CAD build for the part. Positions are in the model's coordinates, mm. A direction names the side the tool comes from. Coordinates: 2 decimals unless noted, no trailing zeros. Order: outer loops, then holes, each group sorted by start corner. A loop starts at its lowest first (then second) coordinate and runs counter-clockwise, first axis right, second up. Notation, with made-up numbers: M -5.5,-37.75 L 31.5,-37.75 A23 cw 31.5,-25.75 Z; hole C 37.25,38.25 d8. An arc over 180 degrees is marked long. Write item = value, one per line.
Autodesk Inventor part; units mm, degrees
ref_plane "YZ Plane" through (0, 0, 0) normal (1, 0, 0) x (0, 1, 0)
ref_plane "XZ Plane" through (0, 0, 0) normal (0, 1, 0) x (-1, 0, 0)
ref_plane "XY Plane" through (0, 0, 0) normal (0, 0, 1) x (1, 0, 0)
sketch "스케치1" plane through (0, 0, 0) normal (0, 0, 1) x (1, 0, 0)
  line L0 (900, -225) -> (-900, -225)
  line L1 (-900, -225) -> (-900, 225)
  line L2 (-900, 225) -> (900, 225)
  line L3 (900, 225) -> (900, -225)
  line L4 (900, -225) -> (-900, 225) construction
  line L5 (-900, -225) -> (900, 225) construction
  point P0 (0, 0)
  dimension "d0" = 1800
  dimension "d1" = 450
extrude "돌출1" add sketch "스케치1" along normal blind 30
sketch "스케치2" plane through (0, 0, 30) normal (0, 0, 1) x (1, 0, 0)
  line L0 (-900, -225) -> (900, -225)
  line L1 (-850, 175) -> (850, 175)
  line L2 (850, 175) -> (850, -225)
  line L3 (850, -225) -> (-850, -225)
  line L4 (-850, -225) -> (-850, 175)
  line L5 (900, 225) -> (-900, 225)
  line L6 (-900, 225) -> (-900, -225)
  line L7 (900, -225) -> (900, 225)
  point P0 (0, 0)
  dimension "d4" = 50
  dimension "d5" = 50
  dimension "d6" = 50
extrude "돌출2" add sketch "스케치2" along normal blind 350 contours L4 L1 L2 L0
sketch "스케치3" plane through (-850, 175, 30) normal (0, 1, 0) x (1, 0, 0)
  line L0 (0, 0) -> (1700, 0) construction
  line L1 (850, 0) -> (850, -673.9117) construction
  line L2 (30, -30) -> (530, -30)
  line L3 (530, -30) -> (530, -150)
  line L4 (530, -150) -> (30, -150)
  line L5 (30, -150) -> (30, -30)
  line L6 (0, 0) -> (0, -350)
  line L7 (1170, -30) -> (1670, -30)
  line L8 (1670, -30) -> (1670, -150)
  line L9 (1670, -150) -> (1170, -150)
  line L10 (1170, -150) -> (1170, -30)
  line L11 (1700, 0) -> (1700, -350)
  line L12 (30, -190) -> (530, -190)
  line L13 (530, -190) -> (530, -310)
  line L14 (530, -310) -> (30, -310)
  line L15 (30, -310) -> (30, -190)
  line L16 (1670, -190) -> (1170, -190)
  line L17 (1170, -190) -> (1170, -310)
  line L18 (1170, -310) -> (1670, -310)
  line L19 (1670, -310) -> (1670, -190)
  point P0 (850, 30)
  dimension "d9" = 120
  dimension "d10" = 30
  dimension "d11" = 120
  dimension "d12" = 30
  dimension "d13" = 500
  dimension "d14" = 500
  dimension "d15" = 120
  dimension "d16" = 40
  dimension "d17" = 30
  dimension "d18" = 30
extrude "돌출3" cut sketch "스케치3" against normal blind 380
sketch "스케치4" plane through (-850, 175, 30) normal (0, 1, 0) x (1, 0, 0)
  line L0 (850, 30) -> (850, -738.9352) construction
  line L1 (1152.4561, -310) -> (547.5439, -310)
  line L2 (547.5439, -310) -> (547.5439, -30)
  line L3 (547.5439, -30) -> (1152.4561, -30)
  line L4 (1152.4561, -30) -> (1152.4561, -310)
  line L5 (1152.4561, -310) -> (547.5439, -30) construction
  line L6 (547.5439, -310) -> (1152.4561, -30) construction
  line L7 (30, -30) -> (530, -30)
  line L8 (530, -310) -> (30, -310)
  point P0 (850, -170)
  dimension "d21" = 0
  dimension "d22" = 0
extrude "돌출4" cut sketch "스케치4" against normal blind 380
sketch "스케치5" plane through (0, 0, 380) normal (0, 0, 1) x (1, 0, 0)
  line L0 (-800, 125) -> (800, 125) construction
  line L1 (800, 125) -> (800, -175) construction
  line L2 (800, -175) -> (-800, -175) construction
  line L3 (-800, -175) -> (-800, 125) construction
  line L4 (850, 175) -> (-850, 175)
  line L5 (-850, -225) -> (850, -225)
  line L6 (850, -225) -> (850, 175)
  line L7 (-850, 175) -> (-850, -225)
  circle A0 centre (-800, 125) radius 25
  circle A1 centre (800, 125) radius 25
  circle A2 centre (800, -175) radius 25
  circle A3 centre (-800, -175) radius 25
  point P0 (0, 0)
  dimension "d26" = 50
  dimension "d27" = 50
  dimension "d28" = 50
  dimension "d29" = 50
  dimension "d30" = 50
  dimension "d31" = 50
  dimension "d32" = 50
  dimension "d33" = 50
extrude "돌출5" add sketch "스케치5" along normal blind 100 contours A0 | A1 | A2 | A3
properties part number "240531_3Dstorage"
(1) Slice it at D-D, the plane y = 125. State how many separate pieces and enclosed holes the cut face has, then the cut area to 3 significant figures.
Evaluation:
separate_pieces = 1
enclosed_holes = 5
area = 250,000 mm²
(2) Slice it at B-B, the plane y = 18. Write the cut outline in (x, z).
Evaluation:
outline = M -900,0 L 900,0 L 900,30 L 850,30 L 850,380 L -850,380 L -850,30 L -900,30 Z; hole M -820,60 L -320,60 L -320,180 L -820,180 Z; hole M -820,220 L -320,220 L -320,340 L -820,340 Z; hole M -302.46,60 L 302.46,60 L 302.46,340 L -302.46,340 Z; hole M 320,60 L 820,60 L 820,180 L 320,180 Z; hole M 320,220 L 820,220 L 820,340 L 320,340 Z
(3) Slice it at A-A, the plane x = -800. Write the cut outline in (y, z), then the cut area to 3 significant figures.
Evaluation:
outline = M -225,0 L 225,0 L 225,30 L 175,30 L 175,60 L -205,60 L -205,180 L 175,180 L 175,220 L -205,220 L -205,340 L 175,340 L 175,380 L 150,380 L 150,480 L 100,480 L 100,380 L -150,380 L -150,480 L -200,480 L -200,380 L -225,380 Z
area = 72,300 mm²
(4) Tool access for faces 5 (the face through (-850, -28, 203)), 6 (the face through (566, -12, 340)), 7 (the face through (900, 3, 15)), 8 (the face through (-786.56, -196.08, 429.3)), 9 (the face through (800, 125, 480)): list every direction of +Z, -Z, +X, -X, +Y, -Y with a clear straight run to the whole face (end or side of a thin tool).
Evaluation:
face_5 = +Z, -X, +Y, -Y
face_6 = +Y
face_7 = +Z, -Z, +X, +Y, -Y
face_8 = +Z
face_9 = +Z, +X, -X, +Y, -Y
(5) Slice it at C-C, the plane x = -426. Write the cut outline in (y, z), then the cut area to 3 significant figures.
Evaluation:
outline = M -225,0 L 225,0 L 225,30 L 175,30 L 175,60 L -205,60 L -205,180 L 175,180 L 175,220 L -205,220 L -205,340 L 175,340 L 175,380 L -225,380 Z
area = 62,300 mm²
(6) Wall check: line 1 (X direction, y = 73, z = 125.5); line 2 (Z direction, x = 701, y = -176); line 3 (Z direction, x = 151, y = 8). Give the ranges that are in metal, low to high. Write a range as from..to.
Evaluation:
line_1 = -850..-820, -320..-302.46, 302.46..320, 820..850
line_2 = 0..60, 180..220, 340..380
line_3 = 0..60, 340..380
(7) Pull direction X, two halves, no side cores. Call faces 1 (the face through (-900, -3, 15)), 2 (the face through (-776.154, 117.491, 429.3)), 3 (the face through (574, -12, 180)), 4 (the face through (-4, 184, 30)): +X half, -X half, draft (parallel to the pull), parting line (faces both ways), or undercut.
Evaluation:
face_1 = -X half
face_2 = undercut
face_3 = undercut
face_4 = draft
(8) Pin check, flat tips, straight feed: pin 1 Ø2 at (y, z) = (47.5, 292.5) entering from -X; pin 2 Ø8 at (y, z) = (104.5, 390.5) entering from -X; pin 3 Ø6 at (x, z) = (636.5, 177.5) entering from +Y. Stop position of each tip, or through.
Evaluation:
pin_1 = -850
pin_2 = -818.78
pin_3 = 175
